Check sheet for the modelled part. Datum: model origin and axes. Units: mm. Face numbers are marked on the shaded views. A direction names the side the tool comes from. Give positions to 0.01 mm unless a question says otherwise; leave off trailing zeros. Loops run counter-clockwise (first coordinate to the right, second up) from the corner with the lowest first, then second, coordinate; pieces in that order, holes last. Notation, with made-up numbers: (-6, -3.5) - (23, -3.5) arc R25 cw to (23, 8.5) - close; hole circle Ø3 at (3, -13). An arc over 180 degrees is marked (long way). Answer in a Markdown table with one row per item. Add a question column.
(1) Go/stop test with flat-tipped pins: P1, Ø2, axis at x = 4, y = 4, coming from the -Z side; P2, Ø3.5, axis at x = 0.5, z = -0.5, coming from the -Y side; P3, Ø2.5, axis at x = 0.5, z = 1, coming from the +Y side. Record where each tip stops, or that it passes through.
(2) Sectioned sample at C-C on z = 0.5. Enter the section's corners in (x, y).
(3) Sectioned sample at B-B on x = 0. Enter the section's corners in (y, z) (3 decimals).
(4) Draft check along X on the marked faces 3, 4, 5 and 6. Enter one of: released by +X, released by -X, zero draft, split by the parting line, or undercut.
(5) Sectioned sample at A-A on y = 8.5. Enter the section's corners in (x, z), then the cut area to 3 significant figures.
(6) Sectioned sample at D-D on y = 3. Enter the section's corners in (x, z) (3 decimals), then the cut area to 3 significant figures.
(7) Set-up check for the marked faces 1 and 2: record each of +Z, -Z, +X, -X, +Y, -Y from which the full face is reachable in a straight line by a thin tool's end or side.
(8) Thickness scan on L1, parallel to Z at x = 0, y = 5 (3 decimals); L2, parallel to Z at x = 0, y = 11.1; L3, parallel to Y at x = 3, z = 2. Record the ranges inside material, lowest first.
Autodesk Inventor part; units mm, degrees
ref_plane "YZ Plane" through (0, 0, 0) normal (1, 0, 0) x (0, 1, 0)
ref_plane "XZ Plane" through (0, 0, 0) normal (0, 1, 0) x (-1, 0, 0)
ref_plane "XY Plane" through (0, 0, 0) normal (0, 0, 1) x (1, 0, 0)
sketch "Sketch1" plane through (0, 0, 0) normal (0, 0, 1) x (1, 0, 0)
  line L0 (0, 0) -> (4.445, 0)
  line L1 (4.445, 0) -> (4.445, 7.2771)
  line L2 (4.445, 7.2771) -> (6.5111, 7.2771)
  line L3 (6.5111, 7.2771) -> (6.5111, 11.176)
  line L4 (6.5111, 11.176) -> (0, 11.176)
  line L5 (0, 11.176) -> (0, 0)
  line L6 (6.5111, 11.176) -> (3.2556, 5.5372) construction
  line L7 (3.2556, 5.5372) -> (-3.2556, 5.5372) construction
  line L8 (-3.2556, 5.5372) -> (-6.5111, 11.176) construction
  line L9 (-6.5111, 11.176) -> (-3.2556, 16.8148) construction
  line L10 (-3.2556, 16.8148) -> (3.2556, 16.8148) construction
  line L11 (3.2556, 16.8148) -> (6.5111, 11.176) construction
  line L12 (3.81, 11.176) -> (3.81, 11.049)
  line L13 (3.81, 11.049) -> (0, 11.049)
  line L14 (3.5179, 0) -> (3.5179, 9.017)
  line L15 (3.5179, 9.017) -> (0, 9.017)
  dimension "d0" = 8.89
  dimension "d2" = 3.8989
  dimension "d3" = 11.2776
  dimension "d7" = 11.176
  dimension "d8" = 7.62
  dimension "d9" = 0.127
  dimension "d10" = 7.0358
  dimension "d11" = 9.017
revolve "Revolution1" add sketch "Sketch1" angle 360 about axis through (0, 11.176, 0) along (0, -1, 0) contours L14 L15 L5 L13 L12 L4 L3 L2 L1 L0
sketch "Sketch2" plane through (0, 11.176, 0) normal (0, 1, 0) x (1, 0, 0)
  line L0 (6.5111, 0) -> (3.2556, -5.6388)
  line L1 (3.2556, -5.6388) -> (-3.2556, -5.6388)
  line L2 (-3.2556, -5.6388) -> (-6.5111, 0)
  line L3 (-6.5111, 0) -> (-3.2556, 5.6388)
  line L4 (-3.2556, 5.6388) -> (3.2556, 5.6388)
  line L5 (3.2556, 5.6388) -> (6.5111, 0)
  circle A0 centre (0, 0) radius 6.5111
extrude "Extrusion1" cut sketch "Sketch2" against normal through all contours A0 L0 | L5 A0 | A0 L1 | L4 A0 | A0 L2 | L3 A0
thread "Thread1"
properties part number "9833K21" material "BRONZE, SAE 841"
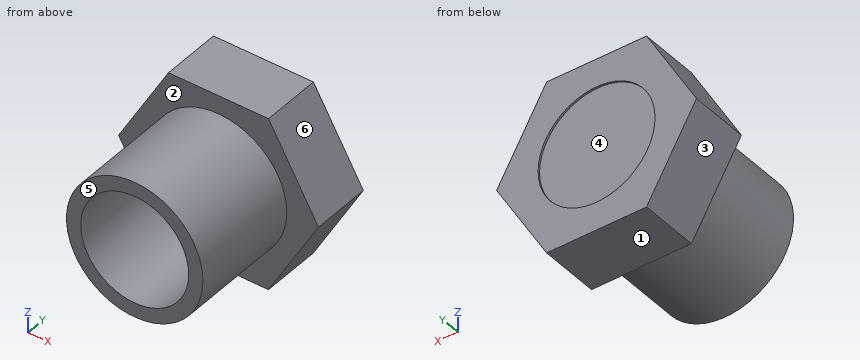
Reply:
| question | item | result |
|---|---|---|
| 1 | P1 | z = -3.28 |
| 1 | P2 | y = 9.02 |
| 1 | P3 | y = 11.05 |
| 2 | outline | (-6.22, 7.28) - (-4.42, 7.28) - (-4.42, 0) - (-3.48, 0) - (-3.48, 9.02) - (3.48, 9.02) - (3.48, 0) - (4.42, 0) - (4.42, 7.28) - (6.22, 7.28) - (6.22, 11.18) - (3.78, 11.18) - (3.78, 11.05) - (-3.78, 11.05) - (-3.78, 11.18) - (-6.22, 11.18) - close |
| 3 | outline | (0, -4.445) - (7.277, -4.445) - (7.277, -5.639) - (11.176, -5.639) - (11.176, -3.81) - (11.049, -3.81) - (11.049, 3.81) - (11.176, 3.81) - (11.176, 5.639) - (7.277, 5.639) - (7.277, 4.445) - (0, 4.445) - (0, 3.518) - (9.017, 3.518) - (9.017, -3.518) - (0, -3.518) - close |
| 4 | face 3 | released by -X |
| 4 | face 4 | undercut |
| 4 | face 5 | zero draft |
| 4 | face 6 | released by +X |
| 5 | outline | (-6.51, 0) - (-3.26, -5.64) - (3.26, -5.64) - (6.51, 0) - (3.26, 5.64) - (-3.26, 5.64) - close; hole circle Ø7.04 at (0, 0) |
| 5 | area | 71.3 mm^2 |
| 6 | outline | circle Ø8.89 at (0, 0); hole circle Ø7.036 at (0, 0) |
| 6 | area | 23.2 mm^2 |
| 7 | face 1 | -Z, +X, -X, +Y, -Y |
| 7 | face 2 | -Y |
| 8 | L1 | -4.445 to -3.518, 3.518 to 4.445 |
| 8 | L2 | -5.64 to -3.81, 3.81 to 5.64 |
| 8 | L3 | 0 to 11.05 |
